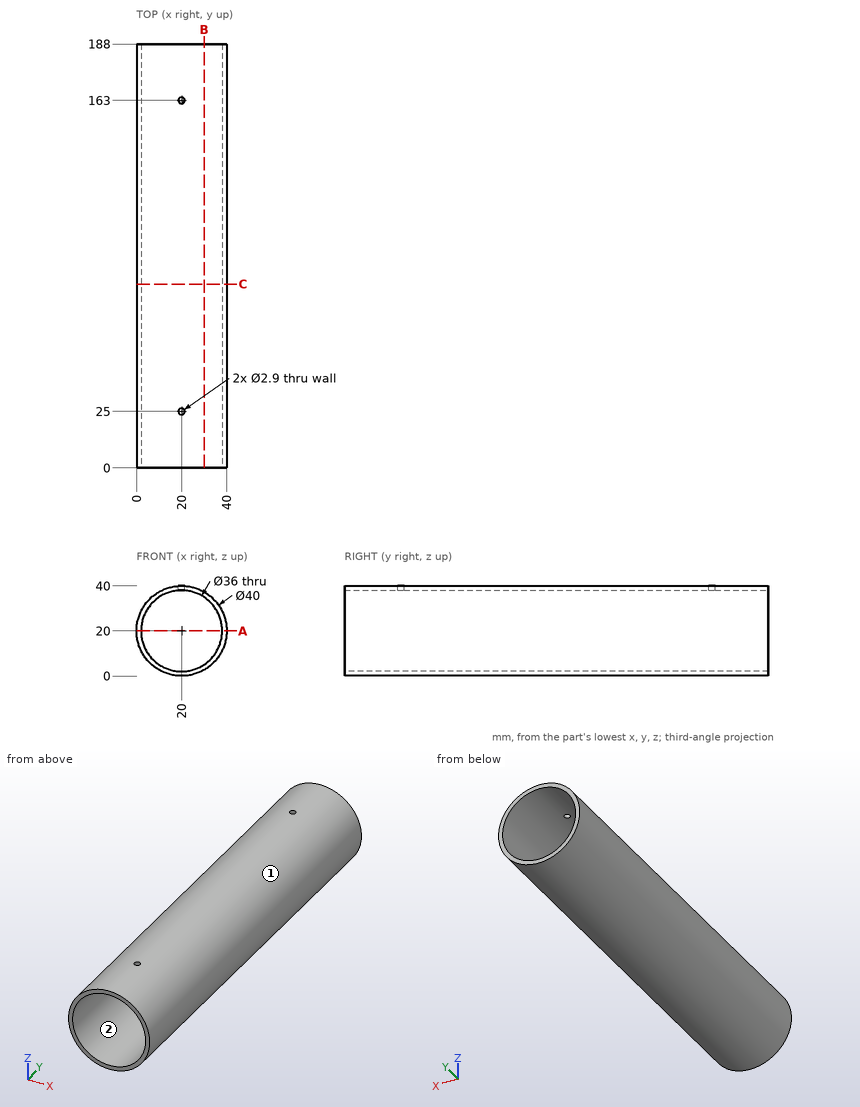
Can you work these out from the drawing? Everything is in mm from the part's minimum corner. Give positions to 0.01 mm unless a question says otherwise; leave off trailing zeros. Loops run counter-clockwise (first coordinate to the right, second up) from the corner with the lowest first, then second, coordinate; pieces in that order, holes last. Notation, with made-up numbers: (28, 74) -> (61, 74) arc R19 ccw to (61, 98) -> close; hole circle Ø9 at (39, -29.5). An arc over 180 degrees is marked (long way). Put each result on its own line as item: value.
(1) Thinking about a two-plate mould opening in Z: for the marked faces 1 and 2, which applies, pulls with the +Z half, pulls with the -Z half, needs draft (parallel to the pull), parting line crosses it, or undercut?
Computed:
face 1: parting line crosses it
face 2: undercut
(2) Imagine slicing it at B-B on x = 30. Write out the boundary of the cut face in (y, z).
Computed:
outline: (0, 2.68) -> (188, 2.68) -> (188, 5.03) -> (0, 5.03) -> close; (0, 34.97) -> (188, 34.97) -> (188, 37.32) -> (0, 37.32) -> close
(3) Imagine slicing it at C-C on y = 81.5. Write out the boundary of the cut face in (x, z).
Computed:
outline: circle Ø40 at (20, 20); hole circle Ø36 at (20, 20)
(4) Please list where these lines run through material, in increasing order: probe 1 along X at (y, z) = (150, 20); probe 2 along Z at (x, y) = (30.5, 128.5); probe 3 along Z at (x, y) = (18, 60). Write a range as [from, to].
Computed:
probe 1: [0, 2], [38, 40]
probe 2: [2.98, 5.38], [34.62, 37.02]
probe 3: [0.1, 2.11], [37.89, 39.9]
(5) I'm going to push flat-ended pins straight in: pin 1 Ø12 at (x, y) = (8, 146) entering from +Z; pin 2 Ø2 at (x, y) = (31.5, 65) entering from +Z; pin 3 Ø1.5 at (y, z) = (84.5, 28) entering from -X. Where does each tip first touch, or does it pass through?
Computed:
pin 1: z = 39.08
pin 2: z = 37.02
pin 3: x = 1.36
(6) Imagine slicing it at A-A on z = 20. Write out the boundary of the cut face in (x, y), plus the area to 3 significant figures.
Computed:
outline: (0, 0) -> (2, 0) -> (2, 188) -> (0, 188) -> close; (38, 0) -> (40, 0) -> (40, 188) -> (38, 188) -> close
area: 752 mm^2
